Autodesk Inventor part; units mm, degrees
ref_plane "YZ Plane" through (0, 0, 0) normal (1, 0, 0) x (0, 1, 0)
ref_plane "XZ Plane" through (0, 0, 0) normal (0, 1, 0) x (-1, 0, 0)
ref_plane "XY Plane" through (0, 0, 0) normal (0, 0, 1) x (1, 0, 0)
sketch "Esboço1" plane through (0, 0, 0) normal (0, 0, 1) x (1, 0, 0)
  line L0 (-10, 10) -> (10, 10)
  line L1 (10, 10) -> (10, -10)
  line L2 (10, -10) -> (-10, -10)
  line L3 (-10, -10) -> (-10, 10)
  line L4 (-10, 10) -> (10, -10) construction
  line L5 (10, 10) -> (-10, -10) construction
  line L6 (-7.5, -7.5) -> (7.5, -7.5)
  line L7 (7.5, -7.5) -> (7.5, 7.5)
  line L8 (7.5, 7.5) -> (-7.5, 7.5)
  line L9 (-7.5, 7.5) -> (-7.5, -7.5)
  line L10 (-7.5, -7.5) -> (7.5, 7.5) construction
  line L11 (7.5, -7.5) -> (-7.5, 7.5) construction
  point P0 (0, 0)
  point P1 (0, 0)
  point P2 (0, 0)
  dimension "d0" = 20
  dimension "d1" = 10
  dimension "d2" = 15
  dimension "d3" = 15
extrude "Extrusão1" add sketch "Esboço1" along normal mid plane 30
sketch "Esboço2" plane through (0, 0, 15) normal (0, 0, 1) x (1, 0, 0)
  line L0 (10, -10) -> (10, 10)
  point P0 (0, 0)
  point P1 (9, 0)
sketch "Esboço10" plane through (0, 0, 0) normal (1, 0, 0) x (0, 1, 0)
  point P0 (0, 0)
sketch "Esboço12" plane through (0, 0, 0) normal (1, 0, 0) x (0, 1, 0)
  line L0 (9, 14) -> (7, 14)
  line L1 (7, 14) -> (7, 12)
  line L2 (7, 12) -> (9, 12)
  line L3 (9, 12) -> (9, 14)
  line L4 (9, 14) -> (7, 12) construction
  line L5 (7, 14) -> (9, 12) construction
  point P0 (0, 0)
  point P1 (8, 13)
properties part number "Peça6_cube"
Source: CAD feature listing. Evaluate the final solid. Frame: model axes, mm. A direction names the side the tool comes from. Give positions to 0.01 mm unless a question says otherwise; leave off trailing zeros. Loops run counter-clockwise (first coordinate to the right, second up) from the corner with the lowest first, then second, coordinate; pieces in that order, holes last. Notation, with made-up numbers: (27.5, 50.25) - (36.5, 50.25) arc R26 ccw to (36.5, 80.25) - close; hole circle Ø5 at (79, 1). An arc over 180 degrees is marked (long way). Use CSV: the item, a comma, the result in double quotes. Start each with the question number.
1. Section C-C (z = -9.5). Output: boundary loops of the cut face in (x, y), then the cut area to 3 significant figures.
2. Section A-A (x = -5.25). Output: boundary loops of the cut face in (y, z).
3. Draft query along Y for faces 3 (the flat face through (10, 0, 0)), 4 (the flat face through (0, -10, 0)), 5 (the flat face through (7.5, 0, 0)). Return one class per face: +Y half, -Y half, draft (parallel to the pull), parting line (faces both ways), or undercut.
4. Reachability of faces 1 (the flat face through (0, 10, 0)), 2 (the flat face through (0, -7.5, 0)) from +Z, -Z, +X, -X, +Y, -Y: full face, straight path, thin tool, end or side. Return the list, or none.
5. Ray query, L1, parallel to Y at x = -5.25, z = 7.75. Return the intervals inside material, ascending.
Response:
1,outline,"(-10, -10) - (10, -10) - (10, 10) - (-10, 10) - close; hole (-7.5, -7.5) - (7.5, -7.5) - (7.5, 7.5) - (-7.5, 7.5) - close"
1,area,"175 mm²"
2,outline,"(-10, -15) - (-7.5, -15) - (-7.5, 15) - (-10, 15) - close; (7.5, -15) - (10, -15) - (10, 15) - (7.5, 15) - close"
3,face 3,"draft"
3,face 4,"-Y half"
3,face 5,"undercut"
4,face 1,"+Z, -Z, +X, -X, +Y"
4,face 2,"+Z, -Z"
5,L1,"-10 to -7.5, 7.5 to 10"
